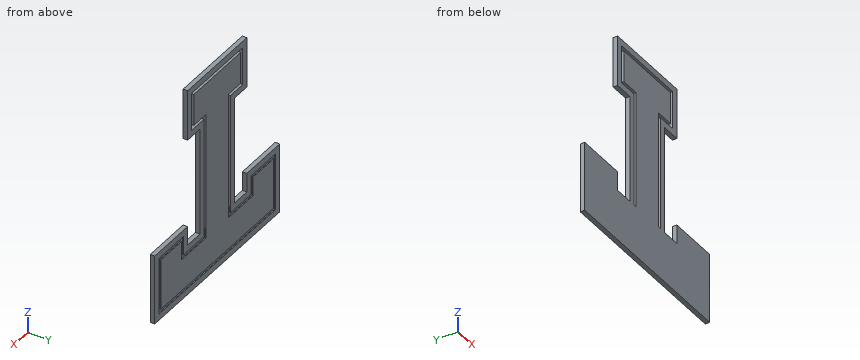
from build123d import *

# Parameters (mm, degrees)
BOSS_EXTRUDE1_DEPTH = 1.778
CUT_EXTRUDE1_DEPTH  = 0.381


with BuildPart() as part:
    # Sketch1 → Boss-Extrude1 (new body)
    with BuildSketch(Plane(origin=(0, 0, 0), x_dir=(1, 0, 0), z_dir=(0, 1, 0))):
        Polygon((-20.32, 83.82), (-20.32, 55.88), (0, 55.88), (0, 63.5), (7.62, 63.5), (7.62, 20.32), (0, 20.32), (0, 0), (36.576, 0), (36.576, 20.32), (28.956, 20.32), (28.956, 63.5), (36.576, 63.5), (36.576, 55.88), (56.896, 55.88), (56.896, 83.82), align=None)
        Polygon((10.16, 17.78), (2.54, 17.78), (2.54, 2.54), (34.036, 2.54), (34.036, 17.78), (26.416, 17.78), (26.416, 63.5), (25.146, 63.5), (25.146, 16.51), (32.766, 16.51), (32.766, 3.81), (3.81, 3.81), (3.81, 16.51), (11.43, 16.51), (11.43, 63.5), (10.16, 63.5), align=None, mode=Mode.SUBTRACT)
    extrude(amount=BOSS_EXTRUDE1_DEPTH)

    # Sketch2 → Cut-Extrude1 (cut)
    with BuildSketch(Plane(origin=(0, 1.778, 0), x_dir=(1, 0, 0), z_dir=(0, 1, 0))):
        Polygon((-16.51, 80.01), (53.086, 80.01), (53.086, 59.69), (40.386, 59.69), (40.386, 67.31), (25.146, 67.31), (25.146, 63.5), (26.416, 63.5), (26.416, 66.04), (39.116, 66.04), (39.116, 58.42), (54.356, 58.42), (54.356, 81.28), (-17.78, 81.28), (-17.78, 58.42), (-2.54, 58.42), (-2.54, 66.04), (10.16, 66.04), (10.16, 63.5), (11.43, 63.5), (11.43, 67.31), (-3.81, 67.31), (-3.81, 59.69), (-16.51, 59.69), align=None)
    extrude(amount=-CUT_EXTRUDE1_DEPTH, mode=Mode.SUBTRACT)


solid = part.part
Work out the finished part from the listing and answer in its coordinate system (mm). Coordinates: 2 decimals unless noted, no trailing zeros. Write each loop counter-clockwise with the first axis right and the second up, starting at its lowest first coordinate (ties: lowest second). Pieces come first, ordered by that corner, then holes. Notation, with made-up numbers: M -19.5,32 L 11.5,32 A20 cw 11.5,55 Z; hole C 72,29 d2. An arc over 180 degrees is marked long. Use one line per item in the form item = value. Start each with the question number.
1. The part is cut by section B-B (x = 20.5). Give the vertices of the cut face in (y, z), plus the area to 3 significant figures.
2. Straight lines are drawn through the part: probe 1 along X at (y, z) = (1.5, -30); probe 2 along Z at (x, y) = (21.5, 1.7); probe 3 along Z at (x, y) = (-3, 1.7). For each, find the intervals that lie inside material, in ascending order. Write a range as from..to.
3. The part is cut by section D-D (x = -9.5). Give the vertices of the cut face in (y, z), plus the area to 3 significant figures.
4. Each of these flat-tipped pins is pushed along its axis until it touches: P1, Ø1.5, axis at x = 29, z = -26.5, coming from the +Y side; P2, Ø0.9, axis at y = 1, z = -9, coming from the -X side; P3, Ø0.5, axis at y = 1, z = -44, coming from the +X side; P4, Ø0.5, axis at y = 0.5, z = -51, coming from the -X side. Where does it stop, or does it pass through?
5. The part is cut by section A-A (z = -33). Give the vertices of the cut face in (x, y).
Evaluation:
q1.outline = M 0,-83.82 L 1.78,-83.82 L 1.78,-81.28 L 1.4,-81.28 L 1.4,-80.01 L 1.78,-80.01 L 1.78,-3.81 L 0,-3.81 Z; M 0,-2.54 L 1.78,-2.54 L 1.78,0 L 0,0 Z
q1.area = 146 mm^2
q2.probe_1 = 7.62..10.16, 11.43..25.15, 26.42..28.96
q2.probe_2 = -83.82..-81.28, -80.01..-3.81, -2.54..0
q2.probe_3 = -83.82..-81.28, -80.01..-67.31, -58.42..-55.88
q3.outline = M 0,-83.82 L 1.78,-83.82 L 1.78,-81.28 L 1.4,-81.28 L 1.4,-80.01 L 1.78,-80.01 L 1.78,-59.69 L 1.4,-59.69 L 1.4,-58.42 L 1.78,-58.42 L 1.78,-55.88 L 0,-55.88 Z
q3.area = 48.7 mm^2
q4.P1 = 1.78
q4.P2 = 0
q4.P3 = 28.96
q4.P4 = 7.62
q5.outline = M 7.62,0 L 10.16,0 L 10.16,1.78 L 7.62,1.78 Z; M 11.43,0 L 25.15,0 L 25.15,1.78 L 11.43,1.78 Z; M 26.42,0 L 28.96,0 L 28.96,1.78 L 26.42,1.78 Z
